Work out the finished part from the listing and answer in its coordinate system (mm). Face numbers are marked on the shaded views. A direction names the side the tool comes from. Give positions to 0.01 mm unless a question says otherwise; leave off trailing zeros. Loops run counter-clockwise (first coordinate to the right, second up) from the corner with the lowest first, then second, coordinate; pieces in that order, holes last. Notation, with made-up numbers: M 63.5,57.25 L 99.5,57.25 A23 ccw 99.5,92.25 Z; hole C 43.25,-12 d1. An arc over 180 degrees is marked long. Use a Markdown table: item, result.
```python
from build123d import *

# Parameters (mm, degrees)
SKETCH1_R           = 1.5
SKETCH1_R_2         = 3
SKETCH1_R_3         = 0.75
SKETCH1_R_4         = 0.5
BOSS_EXTRUDE1_DEPTH = 4


with BuildPart() as part:
    # Sketch1 → Boss-Extrude1 (new body)
    with BuildSketch(Plane.XY):
        with BuildLine():
            Line((16.530619317, 42.42561819), (16.530619317, 22.754982115))
            ThreePointArc((16.530619317, 22.754982115), (22.932240754, 10.915198881), (11.519776525, 3.779592091))
            Line((11.519776525, 3.779592091), (11.147094023, 1.893337277))
            ThreePointArc((11.147094023, 1.893337277), (11.123415667, 1.786594657), (11.094806165, 1.681066709))
            ThreePointArc((11.094806165, 1.681066709), (11.090483266, 1.666641986), (11.086068179, 1.652245212))
            ThreePointArc((11.086068179, 1.652245212), (7.936966432, 0.174837955), (6.754899921, 3.446273846))
            ThreePointArc((6.754899921, 3.446273846), (6.761958039, 3.45957584), (6.769101108, 3.47283241))
            ThreePointArc((6.769101108, 3.47283241), (6.823490663, 3.567681911), (6.882225966, 3.659903468))
            Line((6.882225966, 3.659903468), (7.995950227, 5.322085893))
            ThreePointArc((7.995950227, 5.322085893), (8.251124429, 6.376170558), (7.761765041, 7.344021653))
            ThreePointArc((7.761765041, 7.344021653), (7.549180699, 7.549179572), (7.344022782, 7.761763916))
            ThreePointArc((7.344022782, 7.761763916), (6.376171685, 8.251123307), (5.322087019, 7.995949102))
            Line((5.322087019, 7.995949102), (3.659904592, 6.882224839))
            ThreePointArc((3.659904592, 6.882224839), (3.567683036, 6.823489535), (3.472833536, 6.769099981))
            ThreePointArc((3.472833536, 6.769099981), (3.459576965, 6.761956912), (3.446274971, 6.754898794))
            ThreePointArc((3.446274971, 6.754898794), (0.174839081, 7.936965304), (1.652246338, 11.086067052))
            ThreePointArc((1.652246338, 11.086067052), (1.666643112, 11.090482139), (1.681067834, 11.094805038))
            ThreePointArc((1.681067834, 11.094805038), (1.786595783, 11.12341454), (1.893338403, 11.147092897))
            Line((1.893338403, 11.147092897), (3.856200846, 11.534911383))
            ThreePointArc((3.856200846, 11.534911383), (4.781986668, 12.099826389), (5.120331397, 13.130229803))
            ThreePointArc((5.120331397, 13.130229803), (5.115080125, 13.425618189), (5.120331401, 13.721006575))
            ThreePointArc((5.120331401, 13.721006575), (4.781986671, 14.751409991), (3.856200847, 15.316324996))
            Line((3.856200847, 15.316324996), (1.893338402, 15.704143481))
            ThreePointArc((1.893338402, 15.704143481), (1.786595783, 15.72782184), (1.681067835, 15.756431342))
            ThreePointArc((1.681067835, 15.756431342), (1.666643112, 15.760754241), (1.652246339, 15.765169327))
            ThreePointArc((1.652246339, 15.765169327), (0.174839082, 18.914271075), (3.446274972, 20.096337586))
            ThreePointArc((3.446274972, 20.096337586), (3.459576966, 20.089279467), (3.472833537, 20.082136399))
            ThreePointArc((3.472833537, 20.082136399), (3.567683038, 20.027746844), (3.659904595, 19.969011541))
            Line((3.659904595, 19.969011541), (5.322087019, 18.855287277))
            ThreePointArc((5.322087019, 18.855287277), (6.376171684, 18.600113075), (7.344022779, 19.089472463))
            ThreePointArc((7.344022779, 19.089472463), (7.549180698, 19.302056807), (7.761765042, 19.507214725))
            ThreePointArc((7.761765042, 19.507214725), (8.251124432, 20.475065821), (7.995950227, 21.529150485))
            Line((7.995950227, 21.529150485), (6.882225965, 23.191332912))
            ThreePointArc((6.882225965, 23.191332912), (6.823490661, 23.283554468), (6.769101106, 23.378403968))
            ThreePointArc((6.769101106, 23.378403968), (6.761958038, 23.391660539), (6.754899919, 23.404962533))
            ThreePointArc((6.754899919, 23.404962533), (6.822518946, 25.718097901), (8.837784858, 26.855582349))
            Line((8.837784858, 26.855582349), (10.320619317, 26.855582349))
            Line((10.320619317, 26.855582349), (10.320619317, 42.42561819))
            ThreePointArc((10.320619317, 42.42561819), (13.425619317, 45.53061819), (16.530619317, 42.42561819))
        make_face()
        with Locations((13.425619317, 42.42561819)):
            Circle(SKETCH1_R, mode=Mode.SUBTRACT)
        with Locations((13.425619317, 13.42561819)):
            Circle(SKETCH1_R_2, mode=Mode.SUBTRACT)
        with Locations((11.675619317, 20.42561819)):
            Circle(SKETCH1_R_3, mode=Mode.SUBTRACT)
        with Locations((15.175619317, 20.42561819)):
            Circle(SKETCH1_R_3, mode=Mode.SUBTRACT)
        with Locations((11.675619317, 6.92561819)):
            Circle(SKETCH1_R_4, mode=Mode.SUBTRACT)
        with Locations((15.175619317, 6.92561819)):
            Circle(SKETCH1_R_4, mode=Mode.SUBTRACT)
    extrude(amount=BOSS_EXTRUDE1_DEPTH)


solid = part.part
```
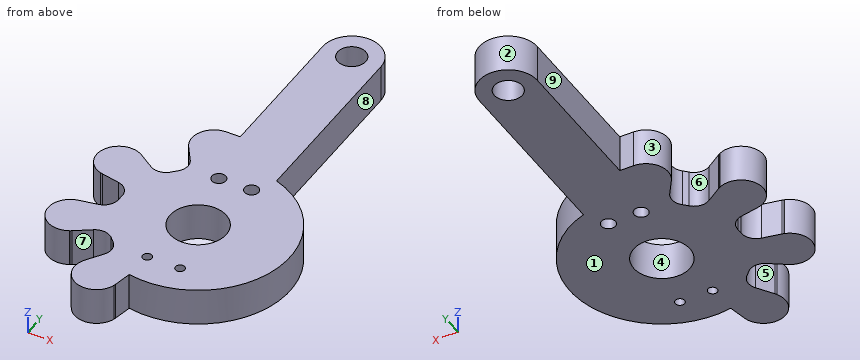
(1) Given P1, Ø1.8, axis at x = 13.43, y = 42.43, coming from the -Z side; P2, Ø1.5, axis at y = 37, z = 1, coming from the +X side; P3, Ø1.5, axis at y = 37.5, z = 0.5, coming from the -X side, each flat-ended and moving along its own axis, determine where each tip first touches the part or whether it passes through.
Entries:
| item | result |
|---|---|
| P1 | passes through |
| P2 | stops at x = 16.53 |
| P3 | stops at x = 10.32 |
(2) The mould has two halves that part along Y. Classify the marked faces 1, 2, 3 and 4: released by +Y, released by -Y, zero draft, split by the parting line, or undercut.
Entries:
| item | result |
|---|---|
| face 1 | zero draft |
| face 2 | released by +Y |
| face 3 | undercut |
| face 4 | undercut |
(3) A cutting plane is placed at C-C (x = 20.75). Write down the section's boundary in (y, z), and give its area (3 significant figures).
Entries:
| item | result |
|---|---|
| outline | M 6.87,0 L 19.99,0 L 19.99,4 L 6.87,4 Z |
| area | 52.5 mm² |
(4) Which of the six approach directions +Z, -Z, +X, -X, +Y, -Y give full straight-line access (tool end or side, diameter ignored) to the marked faces 5, 6, 7, 8 and 9?
Entries:
| item | result |
|---|---|
| face 5 | +Z, -Z, -X |
| face 6 | +Z, -Z |
| face 7 | +Z, -Z, -Y |
| face 8 | +Z, -Z, +X, +Y |
| face 9 | +Z, -Z, -X, +Y |
(5) A cutting plane is placed at A-A (y = 34.5). Write down the section's boundary in (x, z), and give its area (3 significant figures).
Entries:
| item | result |
|---|---|
| outline | M 10.32,0 L 16.53,0 L 16.53,4 L 10.32,4 Z |
| area | 24.8 mm² |
(6) A cutting plane is placed at B-B (z = 2.15). Count the separate pieces of the cut face and the enclosed holes in it, and give its area (3 significant figures).
Entries:
| item | result |
|---|---|
| separate pieces | 1 |
| enclosed holes | 6 |
| area | 456 mm² |
(7) Consider probe 1 along Y at (x, z) = (12.25, 1.15); probe 2 along X at (y, z) = (40, 2.7); probe 3 along Y at (x, z) = (14.25, 2.7). Determine where each line is inside the solid, lowest interval first. Write a range as [from, to].
Entries:
| item | result |
|---|---|
| probe 1 | y = [3.66, 10.67], [16.19, 19.94], [20.91, 41.49], [43.36, 45.3] |
| probe 2 | x = [10.32, 16.53] |
| probe 3 | y = [3.63, 10.54], [16.31, 41.17], [43.68, 45.42] |
